Part print with two shaded views. Sizes in mm from the minimum x, y, z corner. Round coordinates to 2 decimals unless told otherwise and drop trailing zeros. Write each loop counter-clockwise with the first axis right and the second up, starting at its lowest first coordinate (ties: lowest second). Pieces come first, ordered by that corner, then holes. Notation, with made-up numbers: (43.25, 84) -> (93.25, 84) arc R18 ccw to (93.25, 114) -> close; hole circle Ø10 at (16, -17). An arc over 180 degrees is marked (long way). Return JSON: item names as keys, results as strings. Group by question number.
(1) Saw through at C-C (y = 2.6). List the corners of the cut face in (x, z) (1 decimal), plus the area to 3 significant figures.
(2) Drill centre lines: L1, parallel to X at y = 0.3, z = 30.5 (1 decimal); L2, parallel to X at y = 4.65, z = 30. Where is each one in solid material? Low to high. Write a range as from..to.
(3) Saw through at B-B (z = 19.5). List the corners of the cut face in (x, y) (1 decimal).
(4) Mould opens along X. For the marked faces 1 and 2 say: +X half, -X half, draft (parallel to the pull), parting line (faces both ways), or undercut.
(5) Saw through at A-A (x = 14). List the corners of the cut face in (y, z).
(6) Drop flat-ended pins along their axis: pin 1 Ø13 at (x, z) = (29.57, 29.57) entering from +Y; pin 2 Ø2 at (x, y) = (11.5, 1) entering from +Z; pin 3 Ø3 at (y, z) = (1.5, 8) entering from -X. Give the stop position or say it passes through.
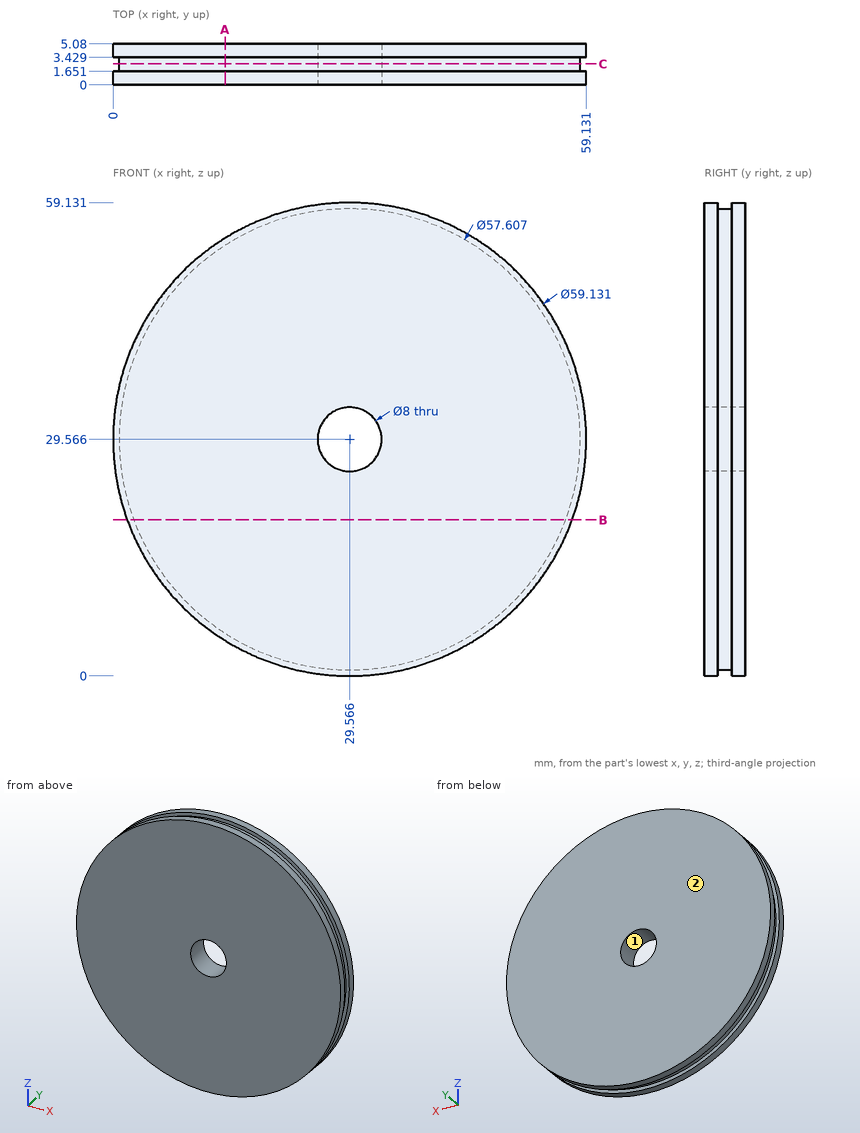
Computed values:
{
 "1": {"outline": "circle Ø57.6 at (29.6, 29.6); hole circle Ø8 at (29.6, 29.6)", "area": "2,560 mm2"},
 "2": {"L1": "0..25.7, 33.5..59.1", "L2": "0..25.59, 33.54..59.13"},
 "3": {"outline": "(1.8, 0) -> (57.4, 0) -> (57.4, 1.7) -> (56.6, 1.7) -> (56.6, 3.4) -> (57.4, 3.4) -> (57.4, 5.1) -> (1.8, 5.1) -> (1.8, 3.4) -> (2.6, 3.4) -> (2.6, 1.7) -> (1.8, 1.7) -> close"},
 "4": {"face 1": "undercut", "face 2": "draft"},
 "5": {"outline": "(0, 4.43) -> (1.65, 4.43) -> (1.65, 5.33) -> (3.43, 5.33) -> (3.43, 4.43) -> (5.08, 4.43) -> (5.08, 54.7) -> (3.43, 54.7) -> (3.43, 53.8) -> (1.65, 53.8) -> (1.65, 54.7) -> (0, 54.7) -> close"},
 "6": {"pin 1": "y = 5.08", "pin 2": "z = 53.71", "pin 3": "x = 7.85"}
}
